For this review, take the finished solid that the model builds, in its own axes (mm). A direction names the side the tool comes from. Give positions to 0.01 mm unless a question says otherwise; leave off trailing zeros. Write each loop counter-clockwise with the first axis right and the second up, starting at its lowest first coordinate (ties: lowest second). Pieces come first, ordered by that corner, then holes.
from build123d import *

# Parameters (mm, degrees)
SKETCH1_R           = 27.85
SKETCH1_R_2         = 22.575
BOSS_EXTRUDE1_DEPTH = 16.4
SKETCH2_R           = 40
SKETCH2_R_2         = 22.575
BOSS_EXTRUDE2_DEPTH = 2.5
SKETCH3_R           = 22.575
SKETCH3_R_2         = 21.5
BOSS_EXTRUDE3_DEPTH = 3
CUT_EXTRUDE1_DEPTH  = 16.4


with BuildPart() as part:
    # Sketch1 → Boss-Extrude1 (new body)
    with BuildSketch(Plane.XY):
        Circle(SKETCH1_R)
        Circle(SKETCH1_R_2, mode=Mode.SUBTRACT)
    extrude(amount=BOSS_EXTRUDE1_DEPTH)

    # Sketch2 → Boss-Extrude2 (add)
    with BuildSketch(Plane.XY.offset(16.4)):
        Circle(SKETCH2_R)
        Circle(SKETCH2_R_2, mode=Mode.SUBTRACT)
    extrude(amount=BOSS_EXTRUDE2_DEPTH)

    # Sketch3 → Boss-Extrude3 (add)
    with BuildSketch(Plane(origin=(0, 0, 0), x_dir=(-1, 0, 0), z_dir=(0, 0, -1))):
        Circle(SKETCH3_R)
        Circle(SKETCH3_R_2, mode=Mode.SUBTRACT)
    extrude(amount=-BOSS_EXTRUDE3_DEPTH)

    # Sketch4 → Cut-Extrude1 (cut)
    with BuildSketch(Plane(origin=(0, 0, 0), x_dir=(-1, 0, 0), z_dir=(0, 0, -1))):
        with BuildLine():
            Line((-15, 21.236760582), (-15, 23.465346791))
            ThreePointArc((-15, 23.465346791), (-27.85, 0), (-15, -23.465346791))
            Line((-15, -23.465346791), (-15, -21.236760582))
            ThreePointArc((-15, -21.236760582), (-26, 0), (-15, 21.236760582))
        make_face()
        with BuildLine():
            ThreePointArc((27.85, 0), (24.427162136, 13.376705499), (15, 23.465346791))
            Line((15, 23.465346791), (15, 21.236760582))
            ThreePointArc((15, 21.236760582), (23.086792761, 11.958260743), (26, 0))
            ThreePointArc((26, 0), (23.086792761, -11.958260743), (15, -21.236760582))
            Line((15, -21.236760582), (15, -23.465346791))
            ThreePointArc((15, -23.465346791), (24.427162136, -13.376705499), (27.85, 0))
        make_face()
    extrude(amount=-CUT_EXTRUDE1_DEPTH, mode=Mode.SUBTRACT)


solid = part.part
(1) Tool access review of faces 4 (the cylindrical face through (-0.22, -27.85, 8.09)), 5 (the flat face through (-20, -8.3, 3)), 6 (the flat face through (26, -8, 16.4)), 7 (the flat face through (-15, 22, 8)): name each direction out of +Z, -Z, +X, -X, +Y, -Y from which nothing blocks a thin tool from reaching the whole face with its end or side.
(2) We need section C-C (y = 9.5). Write out the cut boundary in (x, z), and give its area (3 significant figures).
(3) The part is to be moulded in two halves that separate along X. For faces 1 (the cylindrical face through (2.799, 21.317, 1.479)), 2 (the flat face through (-15, -22, 8)), 3 (the flat face through (17, -17, 18.9)), say which applies: +X half, -X half, draft (parallel to the pull), parting line (faces both ways), or undercut.
(4) We need section A-A (x = 0). Write out the cut boundary in (y, z) (3 decimals).
(5) We need section D-D (y = 25). Write out the cut boundary in (x, z).
(6) Clearance check with flat-ended pins moving along their axes: pin 1 Ø5 at (y, z) = (-8.5, 6) entering from -X; pin 2 Ø24 at (x, y) = (-16.5, -16.5) entering from -Z; pin 3 Ø6 at (y, z) = (17.5, 11) entering from +X; pin 4 Ø0.7 at (y, z) = (-22.5, 12) entering from -X. State where each tip first meets the part, or that it passes through.
(7) We need section B-B (z = 8.5). Write out the cut boundary in (x, y) (3 decimals), and give its area (3 significant figures).
(8) For L1, parallel to Y at x = 0, z = 12 (3 decimals); L2, parallel to X at y = 9.5, z = 7.75; L3, parallel to Y at x = 6.5, z = 17.5, list the stretches that pass through material, from the lowest coordinate up.
The answers:
1. face 4: -Z, -Y
1. face 5: +Z
1. face 6: -Z
1. face 7: -Z, -X, +Y
2. outline: (-38.86, 16.4) - (-24.2, 16.4) - (-24.2, 0) - (-19.29, 0) - (-19.29, 3) - (-20.48, 3) - (-20.48, 18.9) - (-38.86, 18.9) - close; (19.29, 0) - (24.2, 0) - (24.2, 16.4) - (38.86, 16.4) - (38.86, 18.9) - (20.48, 18.9) - (20.48, 3) - (19.29, 3) - close
2. area: 221 mm2
3. face 1: undercut
3. face 2: -X half
3. face 3: draft
4. outline: (-40, 16.4) - (-27.85, 16.4) - (-27.85, 0) - (-21.5, 0) - (-21.5, 3) - (-22.575, 3) - (-22.575, 18.9) - (-40, 18.9) - close; (21.5, 0) - (27.85, 0) - (27.85, 16.4) - (40, 16.4) - (40, 18.9) - (22.575, 18.9) - (22.575, 3) - (21.5, 3) - close
5. outline: (-31.22, 16.4) - (-12.27, 16.4) - (-12.27, 0) - (12.27, 0) - (12.27, 16.4) - (31.22, 16.4) - (31.22, 18.9) - (-31.22, 18.9) - close
6. pin 1: stops at x = -25.3
6. pin 2: stops at z = 0
6. pin 3: stops at x = 21.58
6. pin 4: stops at x = -15
7. outline: (-15, -23.465) arc R27.85 ccw to (15, -23.465) - (15, -21.237) arc R26 ccw to (15, 21.237) - (15, 23.465) arc R27.85 ccw to (-15, 23.465) - (-15, 21.237) arc R26 ccw to (-15, -21.237) - close; hole circle Ø45.15 at (0, 0)
7. area: 640 mm2
8. L1: y = -27.85 to -22.575, 22.575 to 27.85
8. L2: x = -24.2 to -20.48, 20.48 to 24.2
8. L3: y = -39.47 to -21.62, 21.62 to 39.47
